from build123d import *

# Parameters (mm, degrees)
F1_DEPTH = 10
F2_SIZE  = 2


with BuildPart() as f1:
    # F0 (on Top) → F1 (new body)
    with BuildSketch(Plane.XY):
        Polygon((-10, 13), (10, 13), (10, -13), (-10, -13), (-10, -16), (-19, -16), (-19, -13.5), (-21.5, -13.5), (-21.5, -18.5), (-19, -18.5), (-7.5, -18.5), (-7.5, -15.5), (12.5, -15.5), (12.5, 15.5), (-7.5, 15.5), (-7.5, 18.5), (-19, 18.5), (-21.5, 18.5), (-21.5, 13.5), (-19, 13.5), (-19, 16), (-10, 16), align=None)
    extrude(amount=F1_DEPTH)

    # F2
    f2_edges = [f1.edges().sort_by_distance(p)[0] for p in [
        (-19, 13.5, 5),
        (-19, -13.5, 5),
    ]]
    chamfer(f2_edges, length=F2_SIZE)


solid = f1.part
CAD build for the part. Positions are in the model's coordinates, mm. A direction names the side the tool comes from. Give positions to 0.01 mm unless a question says otherwise; leave off trailing zeros. Order: outer loops, then holes, each group sorted by start corner. A loop starts at its lowest first (then second) coordinate and runs counter-clockwise, first axis right, second up. Notation, with made-up numbers: (-23, 8.5) - (13, 8.5) arc R14 ccw to (13, 12.5) - close; hole circle Ø1 at (1, -16). An arc over 180 degrees is marked (long way). Answer in a Markdown table with one row per item.
1. Flat gauge pins, fed straight in: pin 1 (0.9 mm diameter, centred on y = -16.5, z = 4.5, fed in from +X); pin 2 (5 mm diameter, centred on x = 6.5, z = 4.5, fed in from -Y); pin 3 (3 mm diameter, centred on x = 1, z = 3, fed in from +Y). Where does each tip first touch, or does it go through?
Data:
| item | result |
|---|---|
| pin 1 | stops at x = -7.5 |
| pin 2 | stops at y = -15.5 |
| pin 3 | stops at y = 15.5 |
2. Saw through at D-D, the plane y = 16.5. Give the cut face in (x, z), plus the area to 3 significant figures.
Data:
| item | result |
|---|---|
| outline | (-21.5, 0) - (-7.5, 0) - (-7.5, 10) - (-21.5, 10) - close |
| area | 140 mm² |
3. Saw through at C-C, the plane y = -8. Give the cut face in (x, z).
Data:
| item | result |
|---|---|
| outline | (10, 0) - (12.5, 0) - (12.5, 10) - (10, 10) - close |
4. Saw through at A-A, the plane x = -3.5. Give the cut face in (y, z).
Data:
| item | result |
|---|---|
| outline | (-15.5, 0) - (-13, 0) - (-13, 10) - (-15.5, 10) - close; (13, 0) - (15.5, 0) - (15.5, 10) - (13, 10) - close |
5. Saw through at B-B, the plane z = 5. Give the cut face in (x, y).
Data:
| item | result |
|---|---|
| outline | (-21.5, -18.5) - (-7.5, -18.5) - (-7.5, -15.5) - (12.5, -15.5) - (12.5, 15.5) - (-7.5, 15.5) - (-7.5, 18.5) - (-21.5, 18.5) - (-21.5, 13.5) - (-21, 13.5) - (-19, 15.5) - (-19, 16) - (-10, 16) - (-10, 13) - (10, 13) - (10, -13) - (-10, -13) - (-10, -16) - (-19, -16) - (-19, -15.5) - (-21, -13.5) - (-21.5, -13.5) - close |
6. Tool access for faces 1 (the flat face through (-21.5, 16, 5)), 2 (the flat face through (-20, -14.5, 4.9)), 3 (the flat face through (0, -13, 5)), 4 (the flat face through (-7.5, -17, 5)), 5 (the flat face through (-7.5, 17, 5)): list every direction of +Z, -Z, +X, -X, +Y, -Y with a clear straight run to the whole face (end or side of a thin tool).
Data:
| item | result |
|---|---|
| face 1 | +Z, -Z, -X, +Y, -Y |
| face 2 | +Z, -Z |
| face 3 | +Z, -Z, -X |
| face 4 | +Z, -Z, +X, -Y |
| face 5 | +Z, -Z, +X, +Y |
7. Pull direction X, two halves, no side cores. Call faces 6 (the flat face through (-10, 15, 5)), 7 (the flat face through (11, 0, 0)), 8 (the flat face through (-21.5, -16, 5)): pulls with the +X half, pulls with the -X half, needs draft (parallel to the pull), parting line crosses it, or undercut.
Data:
| item | result |
|---|---|
| face 6 | undercut |
| face 7 | needs draft |
| face 8 | pulls with the -X half |
8. Probe probe 1 along Y at (x, z) = (1.5, 1.5); probe 2 along X at (y, z) = (17.5, 1); probe 3 along Y at (x, z) = (-14, 9.25). List the from-to ranges inside material, lowest first. Write a range as [from, to].
Data:
| item | result |
|---|---|
| probe 1 | y = [-15.5, -13], [13, 15.5] |
| probe 2 | x = [-21.5, -7.5] |
| probe 3 | y = [-18.5, -16], [16, 18.5] |
